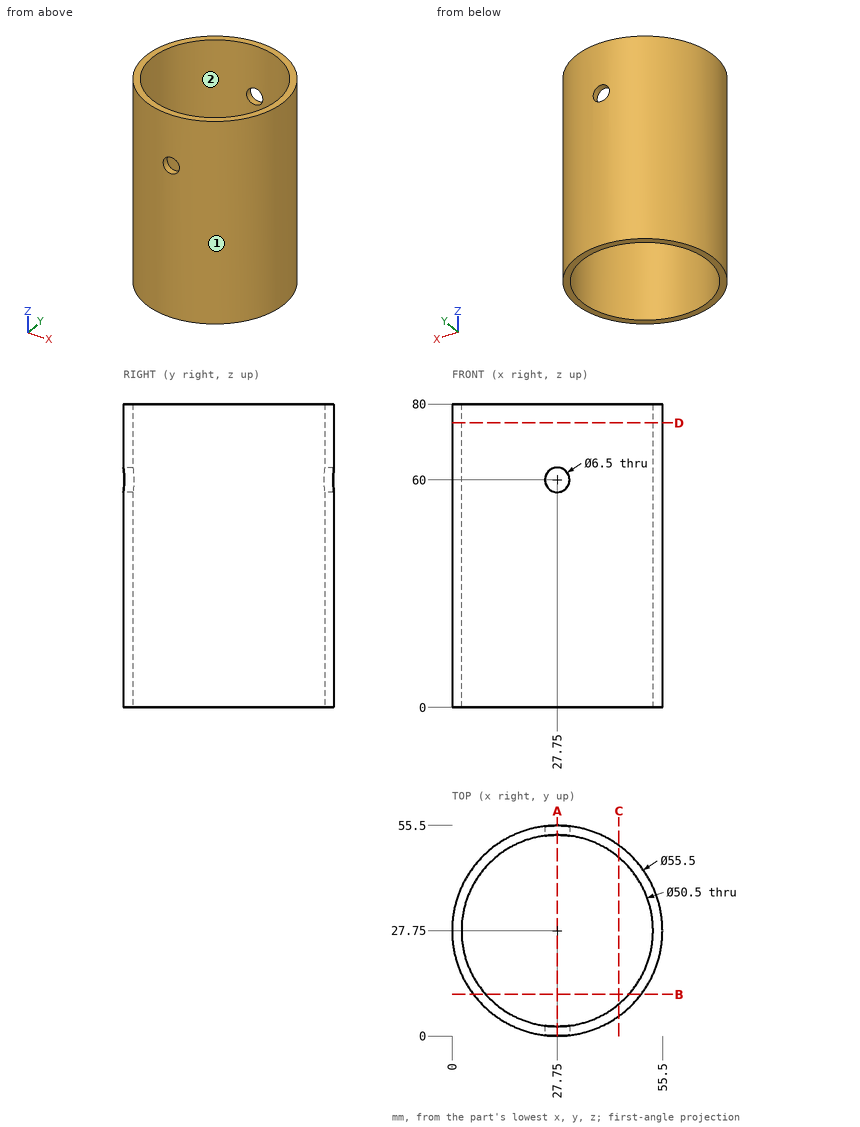
Job drawing, mm, ordinate dimensions from the low corner. One solid piece. Coordinates: 2 decimals unless noted, no trailing zeros. Order: outer loops, then holes, each group sorted by start corner. A loop starts at its lowest first (then second) coordinate and runs counter-clockwise, first axis right, second up. Notation, with made-up numbers: (-5, 83) -> (41, 83) arc R30 cw to (41, 111) -> close; hole circle Ø5 at (75, 32.5). An arc over 180 degrees is marked (long way). Answer in a Markdown table with one row per item. Add a question column.
Q1. Drop flat-ended pins along their axis: pin 1 (1.5 mm diameter, centred on x = 34.5, z = 40.5, fed in from +Y); pin 2 (10 mm diameter, centred on x = 39, z = 13, fed in from -Y); pin 3 (10 mm diameter, centred on y = 33, z = 24.5, fed in from +X); pin 4 (5 mm diameter, centred on x = 27.75, z = 60, fed in from -Y). Give the stop position or say it passes through.
Q2. Wall check: line 1 along Z through (x, y) = (27.75, 1.35); line 2 along Y through (x, z) = (27, 19); line 3 along Y through (x, z) = (26, 55). Give the ranges that are in metal, low to high. Write a range as [from, to].
Q3. Band-saw the part on C-C, the plane x = 44. List the corners of the cut face in (y, z).
Q4. Mould opens along Y. For the marked faces 1 and 2 say: +Y half, -Y half, draft (parallel to the pull), parting line (faces both ways), or undercut.
Q5. Band-saw the part on D-D, the plane z = 75. List the corners of the cut face in (x, y).
Q6. Band-saw the part on B-B, the plane y = 11. List the corners of the cut face in (x, z).
Q7. Band-saw the part on A-A, the plane x = 27.75. List the corners of the cut face in (y, z).
Answers follow:
| question | item | result |
|---|---|---|
| 1 | pin 1 | y = 54.84 |
| 1 | pin 2 | y = 0.71 |
| 1 | pin 3 | x = 55.5 |
| 1 | pin 4 | through |
| 2 | line 1 | [0, 56.75], [63.25, 80] |
| 2 | line 2 | [0.01, 2.51], [52.99, 55.49] |
| 2 | line 3 | [0.06, 2.56], [52.94, 55.44] |
| 3 | outline | (5.26, 0) -> (8.42, 0) -> (8.42, 80) -> (5.26, 80) -> close; (47.08, 0) -> (50.24, 0) -> (50.24, 80) -> (47.08, 80) -> close |
| 4 | face 1 | parting line |
| 4 | face 2 | undercut |
| 5 | outline | circle Ø55.5 at (27.75, 27.75); hole circle Ø50.5 at (27.75, 27.75) |
| 6 | outline | (5.63, 0) -> (8.86, 0) -> (8.86, 80) -> (5.63, 80) -> close; (46.64, 0) -> (49.87, 0) -> (49.87, 80) -> (46.64, 80) -> close |
| 7 | outline | (0, 0) -> (2.5, 0) -> (2.5, 56.75) -> (0, 56.75) -> close; (0, 63.25) -> (2.5, 63.25) -> (2.5, 80) -> (0, 80) -> close; (53, 0) -> (55.5, 0) -> (55.5, 56.75) -> (53, 56.75) -> close; (53, 63.25) -> (55.5, 63.25) -> (55.5, 80) -> (53, 80) -> close |
